Autodesk Inventor part; units mm, degrees
ref_plane "YZ Plane" through (0, 0, 0) normal (1, 0, 0) x (0, 1, 0)
ref_plane "XZ Plane" through (0, 0, 0) normal (0, 1, 0) x (-1, 0, 0)
ref_plane "XY Plane" through (0, 0, 0) normal (0, 0, 1) x (1, 0, 0)
sketch "スケッチ1" plane through (0, 0, 0) normal (0, 0, 1) x (1, 0, 0)
  circle A0 centre (0, 8.5) radius 1.35
  circle A1 centre (0, 0) radius 1.25
  circle A2 centre (0, 0) radius 3
  circle A3 centre (0, 0) radius 6.05
  circle A4 centre (0, 8.5) radius 2.5
  circle A5 centre (-8.5, 0) radius 1.35
  circle A6 centre (-8.5, 0) radius 2.5
  circle A7 centre (0, -8.5) radius 1.35
  circle A8 centre (0, -8.5) radius 2.5
  circle A9 centre (8.5, 0) radius 1.35
  circle A10 centre (8.5, 0) radius 2.5
  circle A11 centre (0, 0) radius 6 construction
  circle A12 centre (0, 0) radius 12
  point P0 (6.0354, -0.4195)
  point P1 (6.0354, 0.4195)
  point P2 (0.4195, 6.0354)
  point P3 (-0.4195, 6.0354)
  point P4 (-6.0354, 0.4195)
  point P5 (-6.0354, -0.4195)
  point P6 (-0.4195, -6.0354)
  point P7 (0.4195, -6.0354)
  dimension "d0" = 2.7
  dimension "d1" = 8.5
  dimension "d3" = 2.5
  dimension "d33" = 6
  dimension "d55" = 12.1
  dimension "d58" = 5
  dimension "d61" = 360
  dimension "d66" = 12
  dimension "d71" = 24
extrude "押し出し1" add sketch "スケッチ1" along normal blind 5 contours A2
extrude "押し出し2" add sketch "スケッチ1" along normal blind 0.45 contours A1 | A2 | A3 A10 | A3 A10 | A4 A3 | A3 A4 | A8 A3 | A3 A8 | A6 A3 | A3 A6
extrude "押し出し3" add sketch "スケッチ1" along normal blind 1.85 contours A12
extrude "押し出し4" add sketch "スケッチ1" along normal blind 1 contours A10 A3 A8 A6 A4
fillet "フィレット2" radius 1 8 edges at (-6.0354, -0.4195, 1.425) (-6.0354, 0.4195, 1.425) (0.4195, -6.0354, 1.425) (-0.4195, -6.0354, 1.425) (6.0354, 0.4195, 1.425) (6.0354, -0.4195, 1.425) (0.4195, 6.0354, 1.425) (-0.4195, 6.0354, 1.425)
properties part number "足首_独立ピッチ_1_2" material "アルミニウム 2014-T4"
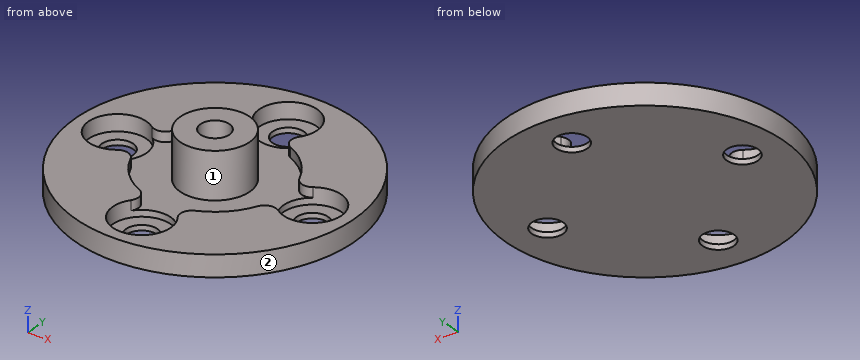
Check sheet for the modelled part. Datum: model origin and axes. Units: mm. Face numbers are marked on the shaded views. A direction names the side the tool comes from. Round coordinates to 2 decimals unless told otherwise and drop trailing zeros. Loops run counter-clockwise (first coordinate to the right, second up) from the corner with the lowest first, then second, coordinate; pieces in that order, holes last.
1. Sectioned sample at D-D on y = -5.25. Record the boundary of the cut face in (x, z).
2. Sectioned sample at B-B on x = -9. Record the boundary of the cut face in (y, z), and give its area (3 significant figures).
3. Sectioned sample at A-A on y = 8.5. Record the boundary of the cut face in (x, z), and give its area (3 significant figures).
4. Sectioned sample at C-C on z = 2.2. Record the boundary of the cut face in (x, y), and give its area (3 significant figures).
5. Gauge pin test, flat ends, axial feed: pin 1 Ø2.5 at (x, y) = (-9, 0.5) entering from +Z; pin 2 Ø3 at (x, z) = (-2, 1.5) entering from +Y; pin 3 Ø8 at (x, y) = (0, 8.5) entering from +Z. Record the tip position at first contact, or that the pin passes through.
6. Set-up check for the marked faces 1 and 2: record each of +Z, -Z, +X, -X, +Y, -Y from which the full face is reachable in a straight line by a thin tool's end or side.
7. Scan lines: probe 1 along Y at (x, z) = (0, 1.3); probe 2 along Y at (x, z) = (0.25, 0.8); probe 3 along Y at (x, z) = (0, 2.65). Record each from-to range of solid material in increasing order.
Recorded:
1. outline: (-10.79, 0) - (10.79, 0) - (10.79, 1.85) - (3.01, 1.85) - (3.01, 1) - (-3.01, 1) - (-3.01, 1.85) - (-10.79, 1.85) - close
2. outline: (-7.94, 0) - (-1.25, 0) - (-1.25, 0.45) - (-2.45, 0.45) - (-2.45, 1.85) - (-7.94, 1.85) - close; (1.25, 0) - (7.94, 0) - (7.94, 1.85) - (2.45, 1.85) - (2.45, 0.45) - (1.25, 0.45) - close
2. area: 21.4 mm2
3. outline: (-8.47, 0) - (-1.35, 0) - (-1.35, 0.45) - (-2.5, 0.45) - (-2.5, 1.85) - (-8.47, 1.85) - close; (1.35, 0) - (8.47, 0) - (8.47, 1.85) - (2.5, 1.85) - (2.5, 0.45) - (1.35, 0.45) - close
3. area: 23.1 mm2
4. outline: circle Ø6 at (0, 0); hole circle Ø2.5 at (0, 0)
4. area: 23.4 mm2
5. pin 1: stops at z = 0.45
5. pin 2: stops at y = 11.99
5. pin 3: stops at z = 1.85
6. face 1: +Z
6. face 2: +Z, -Z
7. probe 1: y = -12 to -11, -3 to -1.25, 1.25 to 3, 11 to 12
7. probe 2: y = -12 to -10.99, -6.01 to -1.22, 1.22 to 6.01, 10.99 to 12
7. probe 3: y = -3 to -1.25, 1.25 to 3
